Could you check a few things on this model? Use its own coordinates, in mm. Face numbers are marked on the shaded views. A direction names the side the tool comes from. Give positions to 0.01 mm unless a question says otherwise; leave off trailing zeros. Loops run counter-clockwise (first coordinate to the right, second up) from the corner with the lowest first, then second, coordinate; pieces in that order, holes last. Notation, with made-up numbers: (81.25, 62.25) - (96.25, 62.25) arc R34 cw to (96.25, 93.25) - close; hole circle Ø2 at (18.25, -20). An arc over 180 degrees is marked (long way). Write each question's results on one line, items separated by ' | '. Start each with the question number.
```python
from build123d import *

# Parameters (mm, degrees)
CUT_EXTRUDE1_REACH     = 32.668
SKETCH4_R              = 1.5
M4_TAPPED_HOLE1_REACH  = 39.835
M4_TAPPED_HOLE1_BORE_R = 1.65


with BuildPart() as part:
    # Sketch1 → Revolve1 (revolve)
    with BuildSketch(Plane(origin=(0, 0, 0), x_dir=(0, 0, -1), z_dir=(1, 0, 0)), mode=Mode.PRIVATE) as revolve1_sk:
        Polygon((6, 0), (6, -14), (20.5, -14), (20.5, -10), (10, -10), (10, 0), align=None)
    revolve(revolve1_sk.sketch.rotate(Axis((0, 12.462470437, 0), (0, -1, 0)), 180), axis=Axis((0, 12.462470437, 0), (0, -1, 0)))

    # Sketch4 → Cut-Extrude1 (cut, up to next)
    with BuildSketch(Plane(origin=(0, -10, 0), x_dir=(1, 0, 0), z_dir=(0, 1, 0)), mode=Mode.PRIVATE) as cut_extrude1_sk1:
        with Locations(Location((0, 15, 0), (0, 0, 270))):
            Circle(SKETCH4_R)
    cut_extrude1_tool1 = extrude(cut_extrude1_sk1.sketch, amount=-CUT_EXTRUDE1_REACH, mode=Mode.PRIVATE) & part.part
    # Sketch4 → Cut-Extrude1 (cut, up to next)
    with BuildSketch(Plane(origin=(0, -10, 0), x_dir=(1, 0, 0), z_dir=(0, 1, 0)), mode=Mode.PRIVATE) as cut_extrude1_sk2:
        with Locations(Location((15, 0, 0), (0, 0, 270))):
            Circle(SKETCH4_R)
    cut_extrude1_tool2 = extrude(cut_extrude1_sk2.sketch, amount=-CUT_EXTRUDE1_REACH, mode=Mode.PRIVATE) & part.part
    # Sketch4 → Cut-Extrude1 (cut, up to next)
    with BuildSketch(Plane(origin=(0, -10, 0), x_dir=(1, 0, 0), z_dir=(0, 1, 0)), mode=Mode.PRIVATE) as cut_extrude1_sk3:
        with Locations(Location((0, -15, 0), (0, 0, 270))):
            Circle(SKETCH4_R)
    cut_extrude1_tool3 = extrude(cut_extrude1_sk3.sketch, amount=-CUT_EXTRUDE1_REACH, mode=Mode.PRIVATE) & part.part
    # Sketch4 → Cut-Extrude1 (cut, up to next)
    with BuildSketch(Plane(origin=(0, -10, 0), x_dir=(1, 0, 0), z_dir=(0, 1, 0)), mode=Mode.PRIVATE) as cut_extrude1_sk4:
        with Locations(Location((-15, 0, 0), (0, 0, 270))):
            Circle(SKETCH4_R)
    cut_extrude1_tool4 = extrude(cut_extrude1_sk4.sketch, amount=-CUT_EXTRUDE1_REACH, mode=Mode.PRIVATE) & part.part
    add(cut_extrude1_tool1.solids().sort_by_distance((0, -10, -15))[0], mode=Mode.SUBTRACT)
    add(cut_extrude1_tool2.solids().sort_by_distance((15, -10, 0))[0], mode=Mode.SUBTRACT)
    add(cut_extrude1_tool3.solids().sort_by_distance((0, -10, 15))[0], mode=Mode.SUBTRACT)
    add(cut_extrude1_tool4.solids().sort_by_distance((-15, -10, 0))[0], mode=Mode.SUBTRACT)

    # M4 Tapped Hole1 bore (on position points) → M4 Tapped Hole1 (cut, up to next)
    with BuildSketch(Plane(origin=(0, -5, -10), x_dir=(-1, 0, 0), z_dir=(0, 0, -1)), mode=Mode.PRIVATE) as m4_tapped_hole1_sk1:
        Circle(M4_TAPPED_HOLE1_BORE_R)
    m4_tapped_hole1_tool1 = extrude(m4_tapped_hole1_sk1.sketch, amount=-M4_TAPPED_HOLE1_REACH, mode=Mode.PRIVATE) & part.part
    add(m4_tapped_hole1_tool1.solids().sort_by_distance((0, -5, -10))[0], mode=Mode.SUBTRACT)


solid = part.part
```
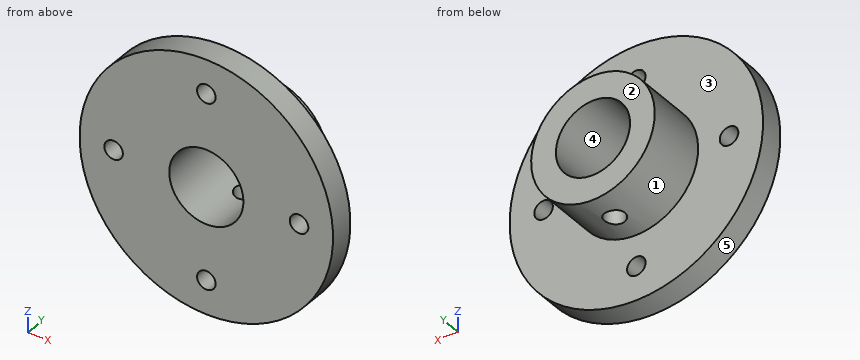
Q1. I want a section at C-C, the plane y = -12.5. List the corners of the cut face in (x, z) for me.
Q2. I want a section at B-B, the plane x = 0. List the corners of the cut face in (y, z) for me, then the cut area to 3 significant figures.
Q3. If we mould it in two halves opening along X, with no side actions, what happens to the marked faces 3, 4 and 5? For each: +X half, -X half, draft (parallel to the pull), parting line (faces both ways), or undercut.
Q4. Which directions (+Z, -Z, +X, -X, +Y, -Y) give clear straight access to the entire face, cutting with the end or side of a thin tool? Please do the marked faces 1 and 2.
Q5. I want a section at A-A, the plane z = 0. List the corners of the cut face in (x, y) for me, then the cut area to 3 significant figures.
Q6. I need wall thicknesses on L1, parallel to X at y = -13.2, z = 0; L2, parallel to X at y = -10.5, z = -1; L3, parallel to X at y = -4, z = 0. Which ranges of each line are inside material? Lowest first, please. Write a range as from..to.
Q7. I want a section at D-D, the plane x = 15. List the corners of the cut face in (y, z) for me, then the cut area to 3 significant figures.
Q8. I'm going to push flat-ended pins straight in: pin 1 Ø2.5 at (x, z) = (0, 15) entering from -Y; pin 2 Ø6 at (y, z) = (-9, -6.5) entering from +X; pin 3 Ø2 at (y, z) = (-12, -5.5) entering from +X; pin 4 Ø5.5 at (x, y) = (0, -5) entering from +Z. Where does each tip first touch, or does it pass through?
Conclusion:
1) outline: circle Ø41 at (0, 0); hole circle Ø3 at (-15, 0); hole circle Ø12 at (0, 0); hole circle Ø3 at (0, -15); hole circle Ø3 at (0, 15); hole circle Ø3 at (15, 0)
2) outline: (-14, -20.5) - (-10, -20.5) - (-10, -16.5) - (-14, -16.5) - close; (-14, -13.5) - (-10, -13.5) - (-10, -10) - (-6.65, -10) - (-6.65, -6) - (-14, -6) - close; (-14, 6) - (0, 6) - (0, 10) - (-10, 10) - (-10, 13.5) - (-14, 13.5) - close; (-14, 16.5) - (-10, 16.5) - (-10, 20.5) - (-14, 20.5) - close; (-3.35, -10) - (0, -10) - (0, -6) - (-3.35, -6) - close | area: 159 mm^2
3) face 3: draft | face 4: undercut | face 5: parting line
4) face 1: +Y | face 2: +Z, -Z, +X, -X, +Y
5) outline: (-20.5, -14) - (-16.5, -14) - (-16.5, -10) - (-20.5, -10) - close; (-13.5, -14) - (-6, -14) - (-6, 0) - (-10, 0) - (-10, -10) - (-13.5, -10) - close; (6, -14) - (13.5, -14) - (13.5, -10) - (10, -10) - (10, 0) - (6, 0) - close; (16.5, -14) - (20.5, -14) - (20.5, -10) - (16.5, -10) - close | area: 172 mm^2
6) L1: -20.5..-16.5, -13.5..-6, 6..13.5, 16.5..20.5 | L2: -20.48..-16.12, -13.88..-5.92, 5.92..13.88, 16.12..20.48 | L3: -10..-6, 6..10
7) outline: (-14, -13.97) - (-10, -13.97) - (-10, -1.5) - (-14, -1.5) - close; (-14, 1.5) - (-10, 1.5) - (-10, 13.97) - (-14, 13.97) - close | area: 99.8 mm^2
8) pin 1: through | pin 2: x = 20.17 | pin 3: x = 20 | pin 4: z = 10
